The listing builds one solid part. Answer for the finished solid, in the listing's coordinates (mm). Face numbers are marked on the shaded views. A direction names the side the tool comes from. Coordinates: 2 decimals unless noted, no trailing zeros. Order: outer loops, then holes, each group sorted by start corner. A loop starts at its lowest first (then second) coordinate and runs counter-clockwise, first axis right, second up. Notation, with made-up numbers: (-9.75, -7) -> (31.25, -7) arc R26 cw to (31.25, 12) -> close; hole circle Ø3 at (22, -8). An arc over 180 degrees is marked (long way). Return JSON: item names as keys, results as strings.
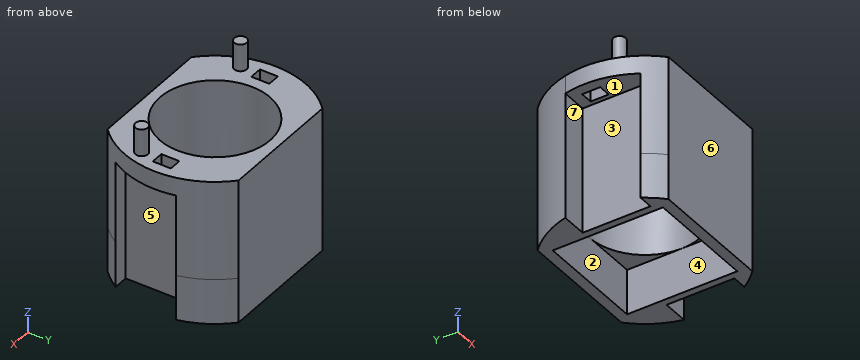
```python
from build123d import *

# Parameters (mm, degrees)
F0_R     = 30.5
F1_DEPTH = 45
F0_R_2   = 3.425
F0_W     = 7
F0_H     = 10
F2_DEPTH = 10
F3_DEPTH = 25
F5_DEPTH = 25


# Not quite as in the source:
# - a feature names something its author has since deleted; it is built from what else it names


with BuildPart() as f1:
    # F0 (on Top) → F1 (new body)
    with BuildSketch(Plane.XY):
        Polygon((34.4299112098, 11.2571539711), (34.4299112098, 36.2571539711), (-34.4299112098, 36.2571539711), (-34.4299112098, 11.2571539711), (-34.4299112098, -26.2571539711), (-34.4299112098, -36.2571539711), (34.4299112098, -36.2571539711), (34.4299112098, -26.2571539711), align=None)
        Circle(F0_R, mode=Mode.SUBTRACT)
        with BuildLine():
            Line((-34.4299112098, 11.2571539711), (-34.4299112098, 36.2571539711))
            ThreePointArc((-34.4299112098, 36.2571539711), (-43.4116633148, 24.8078110329), (-48.7162856186, 11.2571539711))
            Line((-48.7162856186, 11.2571539711), (-34.4299112098, 11.2571539711))
        make_face()
        with BuildLine():
            Line((34.4299112098, 11.2571539711), (48.7162856186, 11.2571539711))
            ThreePointArc((48.7162856186, 11.2571539711), (43.4116633148, 24.8078110329), (34.4299112098, 36.2571539711))
            Line((34.4299112098, 36.2571539711), (34.4299112098, 11.2571539711))
        make_face()
        with BuildLine():
            ThreePointArc((34.4299112098, -36.2571539711), (38.8137028995, -31.5197789844), (42.5506975893, -26.2571539711))
            Line((42.5506975893, -26.2571539711), (34.4299112098, -26.2571539711))
            Line((34.4299112098, -26.2571539711), (34.4299112098, -36.2571539711))
        make_face()
        with BuildLine():
            ThreePointArc((-42.5506975893, -26.2571539711), (-38.8137028995, -31.5197789844), (-34.4299112098, -36.2571539711))
            Line((-34.4299112098, -36.2571539711), (-34.4299112098, -26.2571539711))
            Line((-34.4299112098, -26.2571539711), (-42.5506975893, -26.2571539711))
        make_face()
    extrude(amount=-F1_DEPTH)

    # F0 (on Top) → F2 (join)
    with BuildSketch(Plane.XY):
        Polygon((34.4299112098, 11.2571539711), (34.4299112098, 36.2571539711), (-34.4299112098, 36.2571539711), (-34.4299112098, 11.2571539711), (-34.4299112098, -26.2571539711), (-34.4299112098, -36.2571539711), (34.4299112098, -36.2571539711), (34.4299112098, -26.2571539711), align=None)
        Circle(F0_R, mode=Mode.SUBTRACT)
        with BuildLine():
            Line((-34.4299112098, 11.2571539711), (-48.7162856186, 11.2571539711))
            ThreePointArc((-48.7162856186, 11.2571539711), (-49.3380824624, -8.1088605202), (-42.5506975893, -26.2571539711))
            Line((-42.5506975893, -26.2571539711), (-34.4299112098, -26.2571539711))
            Line((-34.4299112098, -26.2571539711), (-34.4299112098, 11.2571539711))
        make_face()
        with Locations((-40.5626991825, -13.233267504)):
            Circle(F0_R_2, mode=Mode.SUBTRACT)
        with Locations((-40.4299112098, 0.191732496)):
            Rectangle(F0_W, F0_H, mode=Mode.SUBTRACT)
        with BuildLine():
            ThreePointArc((42.5506975893, -26.2571539711), (48.1016365598, -13.6467051066), (50, 0))
            ThreePointArc((50, 0), (49.6780347887, 5.6650560046), (48.7162856186, 11.2571539711))
            Line((48.7162856186, 11.2571539711), (34.4299112098, 11.2571539711))
            Line((34.4299112098, 11.2571539711), (34.4299112098, -26.2571539711))
            Line((34.4299112098, -26.2571539711), (42.5506975893, -26.2571539711))
        make_face()
        with Locations((40.5626991825, -13.233267504)):
            Circle(F0_R_2, mode=Mode.SUBTRACT)
        with Locations((40.4299112098, 0.191732496)):
            Rectangle(F0_W, F0_H, mode=Mode.SUBTRACT)
        with BuildLine():
            Line((34.4299112098, 11.2571539711), (48.7162856186, 11.2571539711))
            ThreePointArc((48.7162856186, 11.2571539711), (43.4116633148, 24.8078110329), (34.4299112098, 36.2571539711))
            Line((34.4299112098, 36.2571539711), (34.4299112098, 11.2571539711))
        make_face()
        with BuildLine():
            Line((-34.4299112098, 11.2571539711), (-34.4299112098, 36.2571539711))
            ThreePointArc((-34.4299112098, 36.2571539711), (-43.4116633148, 24.8078110329), (-48.7162856186, 11.2571539711))
            Line((-48.7162856186, 11.2571539711), (-34.4299112098, 11.2571539711))
        make_face()
        with BuildLine():
            ThreePointArc((34.4299112098, -36.2571539711), (38.8137028995, -31.5197789844), (42.5506975893, -26.2571539711))
            Line((42.5506975893, -26.2571539711), (34.4299112098, -26.2571539711))
            Line((34.4299112098, -26.2571539711), (34.4299112098, -36.2571539711))
        make_face()
        with BuildLine():
            ThreePointArc((-42.5506975893, -26.2571539711), (-38.8137028995, -31.5197789844), (-34.4299112098, -36.2571539711))
            Line((-34.4299112098, -36.2571539711), (-34.4299112098, -26.2571539711))
            Line((-34.4299112098, -26.2571539711), (-42.5506975893, -26.2571539711))
        make_face()
        with Locations((-40.5626991825, -13.233267504)):
            Circle(F0_R_2)
        with Locations((40.5626991825, -13.233267504)):
            Circle(F0_R_2)
    extrude(amount=F2_DEPTH)

    # F0 (on Top) → F3 (join)
    with BuildSketch(Plane.XY):
        with Locations((-40.5626991825, -13.233267504)):
            Circle(F0_R_2)
        with Locations((40.5626991825, -13.233267504)):
            Circle(F0_R_2)
    extrude(amount=F3_DEPTH)

    # F4 (on face) → F5 (join)
    with BuildSketch(Plane(origin=(0, 0, -45), x_dir=(1, 0, 0), z_dir=(0, 0, -1))):
        Polygon((-34.4299112098, -36.2571539711), (34.4299112098, -36.2571539711), (34.4299112098, -11.2571539711), (34.4299112098, 26.2571539711), (34.4299112098, 36.2571539711), (-34.4299112098, 36.2571539711), (-34.4299112098, 26.2571539711), (-34.4299112098, -11.2571539711), align=None)
        Polygon((0, 30.5), (30.5, 30.5), (30.5, 0), (30.5, -30.5), (-3.98e-08, -30.5), (-30.5, -30.5), (-30.5, 4.66e-08), (-30.5, 30.5), align=None, mode=Mode.SUBTRACT)
        with BuildLine():
            Line((34.4299112098, -11.2571539711), (34.4299112098, -36.2571539711))
            ThreePointArc((34.4299112098, -36.2571539711), (43.4116633148, -24.8078110329), (48.7162856186, -11.2571539711))
            Line((48.7162856186, -11.2571539711), (34.4299112098, -11.2571539711))
        make_face()
        with BuildLine():
            ThreePointArc((-48.7162856186, -11.2571539711), (-43.4116633148, -24.8078110329), (-34.4299112098, -36.2571539711))
            Line((-34.4299112098, -36.2571539711), (-34.4299112098, -11.2571539711))
            Line((-34.4299112098, -11.2571539711), (-48.7162856186, -11.2571539711))
        make_face()
        with BuildLine():
            Line((-42.5506975893, 26.2571539711), (-34.4299112098, 26.2571539711))
            Line((-34.4299112098, 26.2571539711), (-34.4299112098, 36.2571539711))
            ThreePointArc((-34.4299112098, 36.2571539711), (-38.8137028995, 31.5197789844), (-42.5506975893, 26.2571539711))
        make_face()
        with BuildLine():
            Line((34.4299112098, 36.2571539711), (34.4299112098, 26.2571539711))
            Line((34.4299112098, 26.2571539711), (42.5506975893, 26.2571539711))
            ThreePointArc((42.5506975893, 26.2571539711), (38.8137028995, 31.5197789844), (34.4299112098, 36.2571539711))
        make_face()
    extrude(amount=F5_DEPTH)


solid = f1.part
```
Item 1: Find the intervals of material crossed by probe 1 along Y at (x, z) = (0, -33); probe 2 along X at (y, z) = (-9.5, -62); probe 3 along Z at (x, y) = (44.5, 5), in increasing order.
Answer list:
{"probe 1": "-36.26 to -30.5, 30.5 to 36.26", "probe 2": "-34.43 to -30.5, 30.5 to 34.43", "probe 3": "0 to 10"}
Item 2: Flat-ended cylindrical pins translate along their axes: pin 1 (4.5 mm diameter, centred on x = -42.5, z = -43, fed in from -Y); pin 2 (7.5 mm diameter, centred on x = 41.5, z = 3.5, fed in from -Y); pin 3 (3 mm diameter, centred on y = 2.5, z = 3.5, fed in from +X); pin 4 (15 mm diameter, centred on x = -19.5, y = -9.5, fed in from -Z). Find the tip coordinate at first contact, or state that the pin passes through.
Answer list:
{"pin 1": "y = -29.66", "pin 2": "y = -32.79", "pin 3": "x = 49.99", "pin 4": "through"}
Item 3: The part is cut by section B-B on z = -48. Determine the outline of the cut face in (x, y).
Answer list:
{"outline": "(-48.72, 11.26) -> (-34.43, 11.26) -> (-34.43, -26.26) -> (-42.55, -26.26) arc R50 ccw to (-34.43, -36.26) -> (34.43, -36.26) arc R50 ccw to (42.55, -26.26) -> (34.43, -26.26) -> (34.43, 11.26) -> (48.72, 11.26) arc R50 ccw to (34.43, 36.26) -> (-34.43, 36.26) arc R50 ccw to start; hole (-30.5, -30.5) -> (30.5, -30.5) -> (30.5, 30.5) -> (-30.5, 30.5) -> close"}
Item 4: Determine the mould class of the marked faces 1, 2 and 3 for opening direction X: pulls with the +X half, pulls with the -X half, needs draft (parallel to the pull), parting line crosses it, or undercut.
Answer list:
{"face 1": "needs draft", "face 2": "undercut", "face 3": "pulls with the -X half"}
Item 5: The part is cut by section C-C on y = 19.5. Determine the outline of the cut face in (x, z), plus the area to 3 significant figures.
Answer list:
{"outline": "(-46.04, -70) -> (-30.5, -70) -> (-30.5, -45) -> (-23.45, -45) -> (-23.45, 10) -> (-46.04, 10) -> close; (23.45, -45) -> (30.5, -45) -> (30.5, -70) -> (46.04, -70) -> (46.04, 10) -> (23.45, 10) -> close", "area": "3,260 mm2"}
Item 6: Which of the six approach directions +Z, -Z, +X, -X, +Y, -Y give full straight-line access (tool end or side, diameter ignored) to the marked faces 4, 5, 6 and 7?
Answer list:
{"face 4": "-Z", "face 5": "-Z, +X", "face 6": "+Z, -Z, +X, -X, -Y", "face 7": "-Z, -X"}
Item 7: The part is cut by section A-A on x = -20. Determine the outline of the cut face in (y, z).
Answer list:
{"outline": "(-36.26, -70) -> (-30.5, -70) -> (-30.5, -45) -> (-23.03, -45) -> (-23.03, 10) -> (-36.26, 10) -> close; (23.03, -45) -> (30.5, -45) -> (30.5, -70) -> (36.26, -70) -> (36.26, 10) -> (23.03, 10) -> close"}
